Could you check a few things on this drawing? It's one solid part, dimensions in mm from its lowest x, y, z. A direction names the side the tool comes from. Coordinates: 2 decimals unless noted, no trailing zeros. Order: outer loops, then holes, each group sorted by start corner. A loop starts at its lowest first (then second) coordinate and runs counter-clockwise, first axis right, second up. Notation, with made-up numbers: M 78.25,12 L 94.25,12 A17 cw 94.25,36 Z; hole C 67,-13.5 d8. An arc over 180 degrees is marked long. Write item = value, one per line. Start each with the question number.
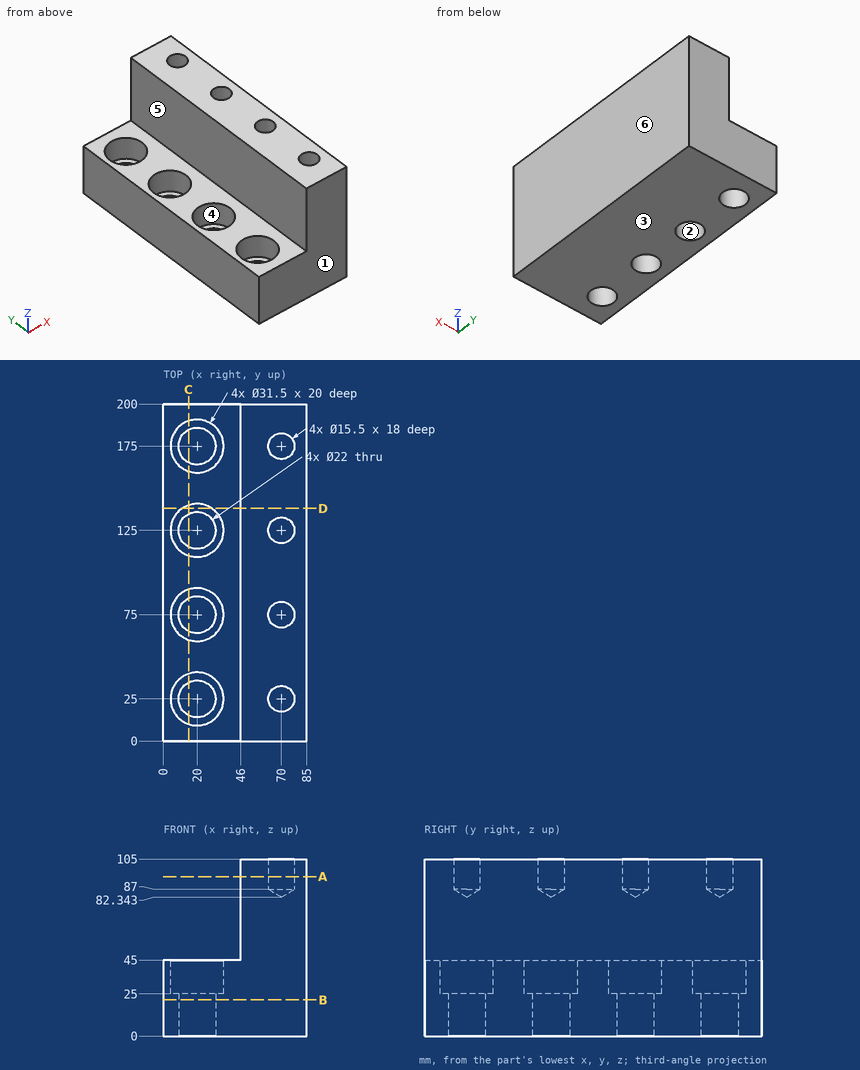
(1) Please list where these lines run through material, in increasing order: probe 1 along Y at (x, z) = (20, 15.75); probe 2 along X at (y, z) = (174.5, 8); probe 3 along Y at (x, z) = (20, 29.75). Write a range as from..to.
(2) Imagine slicing it at B-B on z = 21.5. List the corners of the cut face in (x, y) for me, plus the area to 3 significant figures.
(3) Will these pins go through, and if not, where does the flat tip stop? P1, Ø20, axis at x = 20, y = 125, coming from the -Z side; P2, Ø1.5, axis at x = 39, y = 160.5, coming from the +Z side; P3, Ø4, axis at y = 68, z = 47.5, coming from the -X side; P4, Ø14, axis at x = 70, y = 75, coming from the +Z side.
(4) Imagine slicing it at A-A on z = 94.5. List the corners of the cut face in (x, y) for me.
(5) For the marked faces 4, 5 and 6, which set-ups out of +Z, -Z, +X, -X, +Y, -Y let a thin tool reach every point of the face, with its end or its side?
(6) Thinking about a two-plate mould opening in Y: for the marked faces 1, 2 and 3, which applies, released by +Y, released by -Y, zero draft, split by the parting line, or undercut?
(7) Imagine slicing it at D-D on y = 138. List the corners of the cut face in (x, z) for me.
(8) Imagine slicing it at C-C on x = 15. Give the number of separate pieces and of enclosed holes in the cut face, plus the area to 3 significant figures.
Response:
q1.probe_1 = 0..14, 36..64, 86..114, 136..164, 186..200
q1.probe_2 = 0..9.01, 30.99..85
q1.probe_3 = 0..9.25, 40.75..59.25, 90.75..109.25, 140.75..159.25, 190.75..200
q2.outline = M 0,0 L 85,0 L 85,200 L 0,200 Z; hole C 20,25 d22; hole C 20,75 d22; hole C 20,125 d22; hole C 20,175 d22
q2.area = 15,500 mm2
q3.P1 = through
q3.P2 = 45
q3.P3 = 46
q3.P4 = 86.55
q4.outline = M 46,0 L 85,0 L 85,200 L 46,200 Z; hole C 70,25 d15.5; hole C 70,75 d15.5; hole C 70,125 d15.5; hole C 70,175 d15.5
q5.face_4 = +Z
q5.face_5 = +Z, -X, +Y, -Y
q5.face_6 = +Z, -Z, +X, +Y, -Y
q6.face_1 = released by -Y
q6.face_2 = undercut
q6.face_3 = zero draft
q7.outline = M 0,0 L 85,0 L 85,105 L 46,105 L 46,45 L 28.89,45 L 28.89,25 L 11.11,25 L 11.11,45 L 0,45 Z
q8.separate_pieces = 5
q8.enclosed_holes = 0
q8.area = 4,650 mm2
